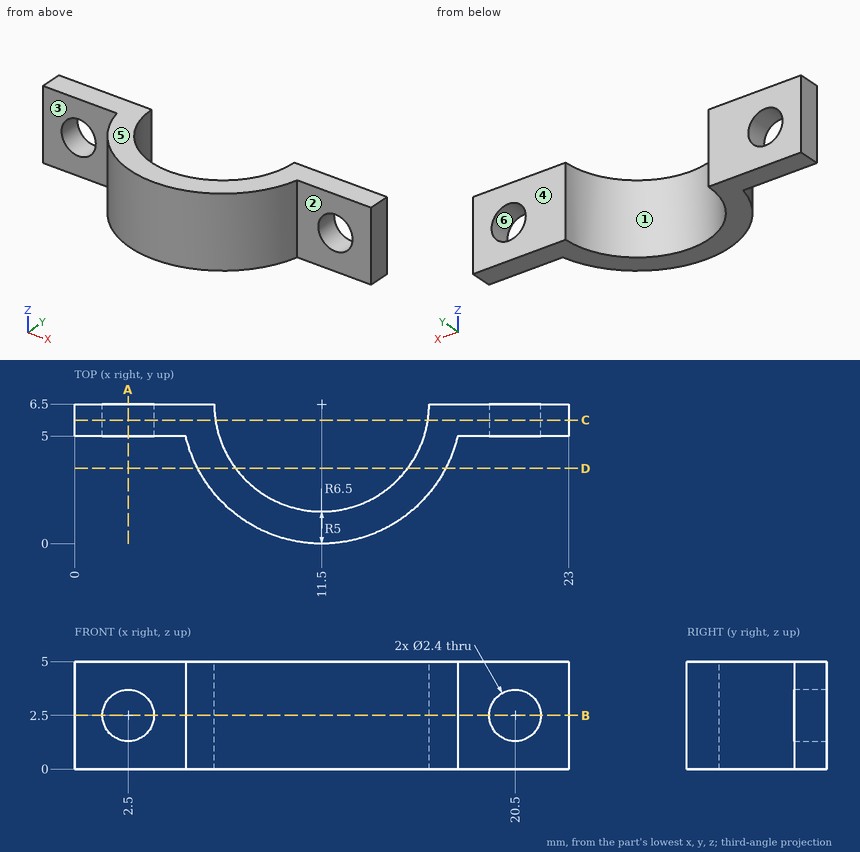
Study the drawing (mm; zero at the part's minimum x, y, z) and answer. A direction names the side the tool comes from. Coordinates: 2 decimals unless noted, no trailing zeros. Write each loop counter-clockwise with the first axis right and the second up, starting at its lowest first coordinate (ties: lowest second). Pieces come first, ordered by that corner, then holes.
Q1. Each of these flat-tipped pins is pushed along its axis until it touches: pin 1 Ø2.5 at (x, z) = (2.5, 2.5) entering from -Y; pin 2 Ø2 at (y, z) = (2.5, 3) entering from -X; pin 3 Ø1.5 at (x, z) = (10.5, 4) entering from -Y; pin 4 Ø2 at (x, z) = (2.5, 2.5) entering from +Y. Where does it stop, or does it pass through?
Q2. Determine the mould class of the marked faces 4, 5 and 6 for opening direction Z: released by +Z, released by -Z, zero draft, split by the parting line, or undercut.
Q3. Which of the six approach directions +Z, -Z, +X, -X, +Y, -Y give full straight-line access (tool end or side, diameter ignored) to the marked faces 1, 2 and 3?
Q4. A cutting plane is placed at A-A, the plane x = 2.5. Give the vertices of the cut face in (y, z).
Q5. A cutting plane is placed at B-B, the plane z = 2.5. Give the vertices of the cut face in (x, y).
Q6. A cutting plane is placed at D-D, the plane y = 3.5. Give the vertices of the cut face in (x, z).
Q7. Find the intervals of material crossed by line 1 (Z direction, x = 20.5, y = 6.1); line 2 (Y direction, x = 19.25, z = 0.85); line 3 (X direction, y = 3.25, z = 4.8), in increasing order.
Q8. A cutting plane is placed at C-C, the plane y = 5.75. Give the vertices of the cut face in (x, z).
Findings below:
1. pin 1: stops at y = 5
1. pin 2: stops at x = 5.73
1. pin 3: stops at y = 0
1. pin 4: passes through
2. face 4: zero draft
2. face 5: released by +Z
2. face 6: undercut
3. face 1: +Z, -Z, +Y
3. face 2: +Z, -Z, +X, -Y
3. face 3: +Z, -Z, -X, -Y
4. outline: (5, 0) - (6.5, 0) - (6.5, 1.3) - (5, 1.3) - close; (5, 3.7) - (6.5, 3.7) - (6.5, 5) - (5, 5) - close
5. outline: (0, 5) - (1.3, 5) - (1.3, 6.5) - (0, 6.5) - close; (3.7, 5) - (5.18, 5) arc R6.5 ccw to (17.82, 5) - (19.3, 5) - (19.3, 6.5) - (16.5, 6.5) arc R5 cw to (6.5, 6.5) - (3.7, 6.5) - close; (21.7, 5) - (23, 5) - (23, 6.5) - (21.7, 6.5) - close
6. outline: (5.73, 0) - (7.5, 0) - (7.5, 5) - (5.73, 5) - close; (15.5, 0) - (17.27, 0) - (17.27, 5) - (15.5, 5) - close
7. line 1: z = 0 to 1.3, 3.7 to 5
7. line 2: y = 5 to 6.5
7. line 3: x = 5.87 to 7.7, 15.3 to 17.13
8. outline: (0, 0) - (6.56, 0) - (6.56, 5) - (0, 5) - close; (16.44, 0) - (23, 0) - (23, 5) - (16.44, 5) - close; hole circle Ø2.4 at (2.5, 2.5); hole circle Ø2.4 at (20.5, 2.5)
